```python
from build123d import *

# Parameters (mm, degrees)
BOSS_EXTRUDE1_DEPTH = 70
FILLET3_R           = 0.5
FILLET4_R           = 0.5
SKETCH2_W           = 5
SKETCH2_H           = 5
CUT_EXTRUDE1_DEPTH  = 5
SKETCH3_R           = 2
CUT_EXTRUDE2_DEPTH  = 73.972597597


with BuildPart() as part:
    # Sketch1 → Boss-Extrude1 (new body)
    with BuildSketch(Plane.XY):
        Polygon((0, 0), (20, 0), (20, 3.5), (13.5, 3.5), (13.5, 5.5), (16.5, 9), (3.5, 9), (6.5, 5.5), (6.5, 3.5), (0, 3.5), align=None)
    extrude(amount=BOSS_EXTRUDE1_DEPTH)

    # Fillet3
    fillet3_edges = [part.edges().sort_by_distance(p)[0] for p in [
        (16.5, 9, 35),
    ]]
    fillet(fillet3_edges, radius=FILLET3_R)

    # Fillet4
    fillet4_edges = [part.edges().sort_by_distance(p)[0] for p in [
        (3.5, 9, 35),
    ]]
    fillet(fillet4_edges, radius=FILLET4_R)

    # Sketch2 → Cut-Extrude1 (cut)
    with BuildSketch(Plane(origin=(0, 9, 0), x_dir=(1, 0, 0), z_dir=(0, 1, 0))):
        with Locations((10, -9.5)):
            Rectangle(SKETCH2_W, SKETCH2_H)
        with Locations((10, -60.5)):
            Rectangle(SKETCH2_W, SKETCH2_H)
    extrude(amount=-CUT_EXTRUDE1_DEPTH, mode=Mode.SUBTRACT)

    # Sketch3 → Cut-Extrude2 (cut, through all)
    with BuildSketch(Plane(origin=(0, 4, 0), x_dir=(1, 0, 0), z_dir=(0, 1, 0))):
        with Locations(Location((10, -9.5, 0), (0, 0, 270))):
            Circle(SKETCH3_R)
        with Locations(Location((10, -60.5, 0), (0, 0, 270))):
            Circle(SKETCH3_R)
    extrude(amount=-CUT_EXTRUDE2_DEPTH, mode=Mode.SUBTRACT)


solid = part.part
```
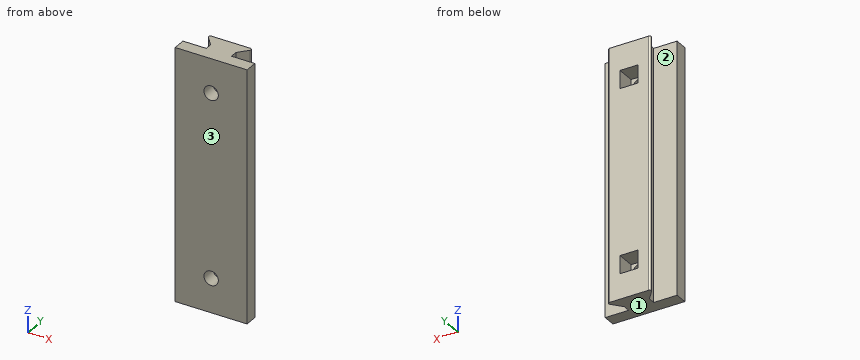
The listing builds one solid part. Answer for the finished solid, in the listing's coordinates (mm). Face numbers are marked on the shaded views. Round coordinates to 2 decimals unless told otherwise and drop trailing zeros. Loops run counter-clockwise (first coordinate to the right, second up) from the corner with the lowest first, then second, coordinate; pieces in that order, holes last. Notation, with made-up numbers: (62, 86.25) - (73, 86.25) arc R28 ccw to (73, 108.25) - close; hole circle Ø8 at (64.25, 44). An arc over 180 degrees is marked (long way). Return JSON: item names as keys, results as strings. Group by question number.
1. Consider probe 1 along X at (y, z) = (2.95, 60.5); probe 2 along X at (y, z) = (4.5, 32); probe 3 along Y at (x, z) = (5.5, 25). Determine where each line is inside the solid, lowest interval first.
2. The part is cut by section C-C on y = 1.5. Determine the outline of the cut face in (x, z), then the cut area to 3 significant figures.
3. The part is cut by section A-A on x = 10. Determine the outline of the cut face in (y, z).
4. Each of these flat-tipped pins is pushed along its axis until it touches: P1, Ø8, axis at x = 11, z = 40.5, coming from the -Y side; P2, Ø4, axis at y = 6, z = 8.5, coming from the +X side; P3, Ø3, axis at x = 10, z = 60.5, coming from the +Y side; P4, Ø1.5, axis at y = 7.5, z = 59.5, coming from the -X side. Where does it stop, or does it pass through?
5. The part is cut by section D-D on z = 23. Determine the outline of the cut face in (x, y), then the cut area to 3 significant figures.
6. The mould has two halves that part along Y. Classify the marked faces 1, 2 and 3: pulls with the +Y half, pulls with the -Y half, needs draft (parallel to the pull), parting line crosses it, or undercut.
7. The part is cut by section B-B on z = 60.5. Determine the outline of the cut face in (x, y), then the cut area to 3 significant figures.
Resolved:
{
 "1": {"probe 1": "x = 0 to 8, 12 to 20", "probe 2": "x = 6.5 to 13.5", "probe 3": "y = 0 to 3.5, 6.67 to 9"},
 "2": {"outline": "(0, 0) - (20, 0) - (20, 70) - (0, 70) - close; hole circle Ø4 at (10, 9.5); hole circle Ø4 at (10, 60.5)", "area": "1,370 mm²"},
 "3": {"outline": "(0, 0) - (9, 0) - (9, 7) - (4, 7) - (4, 7.5) - (0, 7.5) - close; (0, 11.5) - (4, 11.5) - (4, 12) - (9, 12) - (9, 58) - (4, 58) - (4, 58.5) - (0, 58.5) - close; (0, 62.5) - (4, 62.5) - (4, 63) - (9, 63) - (9, 70) - (0, 70) - close"},
 "4": {"P1": "stops at y = 0", "P2": "stops at x = 15.64", "P3": "passes through", "P4": "stops at x = 4.15"},
 "5": {"outline": "(0, 0) - (20, 0) - (20, 3.5) - (13.5, 3.5) - (13.5, 5.5) - (15.79, 8.17) arc R0.5 ccw to (15.41, 9) - (4.59, 9) arc R0.5 ccw to (4.21, 8.17) - (6.5, 5.5) - (6.5, 3.5) - (0, 3.5) - close", "area": "118 mm²"},
 "6": {"face 1": "needs draft", "face 2": "undercut", "face 3": "pulls with the -Y half"},
 "7": {"outline": "(0, 0) - (8, 0) - (8, 4) - (7.5, 4) - (7.5, 9) - (4.59, 9) arc R0.5 ccw to (4.21, 8.17) - (6.5, 5.5) - (6.5, 3.5) - (0, 3.5) - close; (12, 0) - (20, 0) - (20, 3.5) - (13.5, 3.5) - (13.5, 5.5) - (15.79, 8.17) arc R0.5 ccw to (15.41, 9) - (12.5, 9) - (12.5, 4) - (12, 4) - close", "area": "77.5 mm²"}
}
